```python
from build123d import *

# Parameters (mm, degrees)
SKETCH1_R                = 0.95
BOSS_EXTRUDE1_DEPTH      = 2.625
CUT_EXTRUDE1_DEPTH       = 20.729120518
CUT_EXTRUDE1_DEPTH_BACK  = 5.25
SKETCH2_W                = 38
SKETCH2_H                = 2.75
BOSS_EXTRUDE2_DEPTH      = 2.625
BOSS_EXTRUDE2_DEPTH_BACK = 1.375


with BuildPart() as part:
    # Sketch1 → Boss-Extrude1 (new, symmetric)
    with BuildSketch(Plane(origin=(0, 0, 0), x_dir=(1, 0, 0), z_dir=(0, 1, 0))):
        with BuildLine():
            Line((-0.393995074, 3.318856737), (-17.15759803, 1.993781046))
            ThreePointArc((-17.15759803, 1.993781046), (-18.998616533, 0.074377097), (-17.305351185, -1.97655272))
            Line((-17.305351185, -1.97655272), (-0.381688981, -4.591034114))
            ThreePointArc((-0.381688981, -4.591034114), (0, -4.620343214), (0.381688981, -4.591034114))
            Line((0.381688981, -4.591034114), (17.305351185, -1.97655272))
            ThreePointArc((17.305351185, -1.97655272), (18.998616533, 0.074377097), (17.15759803, 1.993781046))
            Line((17.15759803, 1.993781046), (0.393995074, 3.318856737))
            ThreePointArc((0.393995074, 3.318856737), (0, 3.334404121), (-0.393995074, 3.318856737))
        make_face()
        with Locations(Location((-17, 0, 0), (0, 0, 90))):
            Circle(SKETCH1_R, mode=Mode.SUBTRACT)
        with Locations(Location((17, 0, 0), (0, 0, 90))):
            Circle(SKETCH1_R, mode=Mode.SUBTRACT)
        with Locations(Location((0, -1.75, 0), (0, 0, 90))):
            Circle(SKETCH1_R, mode=Mode.SUBTRACT)
    extrude(amount=BOSS_EXTRUDE1_DEPTH, both=True)

    # Sketch2 → Cut-Extrude1 (cut, two sides: drawn at the far end of the back side and taken through both)
    with BuildSketch(Plane.XY.offset(-CUT_EXTRUDE1_DEPTH_BACK)):
        Rectangle(SKETCH2_W, SKETCH2_H)
    extrude(amount=CUT_EXTRUDE1_DEPTH + CUT_EXTRUDE1_DEPTH_BACK, mode=Mode.SUBTRACT)


with BuildPart() as cut_extrude1_piece_1:
    # of the separate pieces the step leaves, piece 1, a body of its own (cut_extrude1_pieces)
    add(part.part.solids().sort_by_distance((17.15759803, 2.625, -1.993781046))[0])



with BuildPart() as cut_extrude1_piece_2:
    # of the separate pieces the step leaves, piece 2, a body of its own (cut_extrude1_pieces)
    add(part.part.solids().sort_by_distance((17.15759803, -1.375, -1.993781046))[0])


with BuildPart() as cut_extrude1_piece_1_1:
    add(cut_extrude1_piece_1.part)

    add(cut_extrude1_piece_2.part)  # Boss-Extrude2 merges Cut-Extrude1 piece 2
    # Sketch3 → Boss-Extrude2 (add, two sides: drawn at the far end of the back side and taken through both)
    with BuildSketch(Plane(origin=(0, 0, 0), x_dir=(1, 0, 0), z_dir=(0, 1, 0)).offset(-BOSS_EXTRUDE2_DEPTH_BACK)):
        with BuildLine():
            Line((12.412535452, -0.081023287), (7.279310345, -2.781023287))
            ThreePointArc((7.279310345, -2.781023287), (6.468976713, -2.529310345), (6.720689655, -1.718976713))
            Line((6.720689655, -1.718976713), (11.853914762, 0.981023287))
            ThreePointArc((11.853914762, 0.981023287), (12.664248394, 0.729310345), (12.412535452, -0.081023287))
        make_face()
    extrude(amount=BOSS_EXTRUDE2_DEPTH + BOSS_EXTRUDE2_DEPTH_BACK)


solid = cut_extrude1_piece_1_1.part
```
Work out the finished part from the listing and answer in its coordinate system (mm). A direction names the side the tool comes from. Give positions to 0.01 mm unless a question says otherwise; leave off trailing zeros. Loops run counter-clockwise (first coordinate to the right, second up) from the corner with the lowest first, then second, coordinate; pieces in that order, holes last. Notation, with made-up numbers: (30.25, 19.25) - (41.25, 19.25) arc R31 cw to (41.25, 52.25) - close; hole circle Ø3 at (11.25, 12). An arc over 180 degrees is marked (long way). One line per question, with ' | ' between items.
(1) The part is cut by section B-B (y = 2). Write down the section's boundary in (x, z).
Recorded:
outline: (-17.31, 1.98) arc R2 ccw to (-17.16, -1.99) - (-0.39, -3.32) arc R5 ccw to (0.39, -3.32) - (17.16, -1.99) arc R2 ccw to (17.31, 1.98) - (0.38, 4.59) arc R2.5 ccw to (-0.38, 4.59) - close; hole circle Ø1.9 at (-17, 0); hole circle Ø1.9 at (0, 1.75); hole circle Ø1.9 at (17, 0)
(2) The mould has two halves that part along Y. Classify faces 3 (the face through (9.882, -0.019, 1.412)), 4 (the face through (17.84, -2.01, -0.44)), 5 (the face through (-0.3, 2.625, 0.6)): +Y half, -Y half, draft (parallel to the pull), parting line (faces both ways), or undercut.
Recorded:
face 3: undercut | face 4: draft | face 5: +Y half
(3) Straight lines are drawn through the part: probe 1 along X at (y, z) = (-2.3, 0); probe 2 along Y at (x, z) = (-3.5, -3) (3 decimals); probe 3 along X at (y, z) = (-2.25, 1.75). For each, find the intervals that lie inside material, in ascending order.
Recorded:
probe 1: x = -19 to -17.95, -16.05 to 16.05, 17.95 to 19 | probe 2: y = -2.625 to -1.375, 1.375 to 2.625 | probe 3: x = -17.97 to -0.95, 0.95 to 17.97
(4) A tool of negligible diameter and unlimited length cuts with its end or side. For faces 1 (the face through (9.25, -0.02, 0.39)), 2 (the face through (8.73, -1.99, 3.3)), from which of +Z, -Z, +X, -X, +Y, -Y can it reach the whole face along a straight path? Write none if from no direction.
Recorded:
face 1: -Z, -X | face 2: +Z, +X, +Y, -Y
(5) The part is cut by section A-A (x = 0). Write down the section's boundary in (y, z) (3 decimals).
Recorded:
outline: (-2.625, -3.334) - (-1.375, -3.334) - (-1.375, 0.8) - (-2.625, 0.8) - close; (-2.625, 2.7) - (-1.375, 2.7) - (-1.375, 4.62) - (-2.625, 4.62) - close; (1.375, -3.334) - (2.625, -3.334) - (2.625, 0.8) - (1.375, 0.8) - close; (1.375, 2.7) - (2.625, 2.7) - (2.625, 4.62) - (1.375, 4.62) - close
(6) The part is cut by section C-C (z = 4). Write down the section's boundary in (x, y) (3 decimals), then the cut area to 3 significant figures.
Recorded:
outline: (-4.207, -2.625) - (4.207, -2.625) - (4.207, -1.375) - (-4.207, -1.375) - close; (-4.207, 1.375) - (4.207, 1.375) - (4.207, 2.625) - (-4.207, 2.625) - close | area: 21.0 mm²
(7) Each of these flat-tipped pins is pushed along its axis until it touches: pin 1 Ø2 at (y, z) = (1, 2) entering from -X; pin 2 Ø1.1 at (x, z) = (0, 1.75) entering from -Y; pin 3 Ø3 at (x, y) = (6, -1.5) entering from +Z; pin 4 Ø3 at (x, y) = (-13.5, -1) entering from +Z. Where does it stop, or does it pass through?
Recorded:
pin 1: stops at x = -18.69 | pin 2: passes through | pin 3: stops at z = 3.95 | pin 4: stops at z = 2.79
(8) The part is cut by section D-D (x = 15.5). Write down the section's boundary in (y, z) (3 decimals).
Recorded:
outline: (-2.625, -2.125) - (-1.375, -2.125) - (-1.375, 2.255) - (-2.625, 2.255) - close; (1.375, -2.125) - (2.625, -2.125) - (2.625, 2.255) - (1.375, 2.255) - close
